Read the model definition and answer for the solid it produces. Units are mm, in the model's axes. Face numbers are marked on the shaded views. A direction names the side the tool comes from. Coordinates: 2 decimals unless noted, no trailing zeros. Write each loop counter-clockwise with the first axis right and the second up, starting at its lowest first coordinate (ties: lowest second). Pieces come first, ordered by that corner, then holes. Notation, with made-up numbers: (77.25, 82) - (120.25, 82) arc R18 cw to (120.25, 103) - close; hole circle Ø2 at (10.5, 40.5). An arc over 180 degrees is marked (long way). Use a Markdown table: item, result.
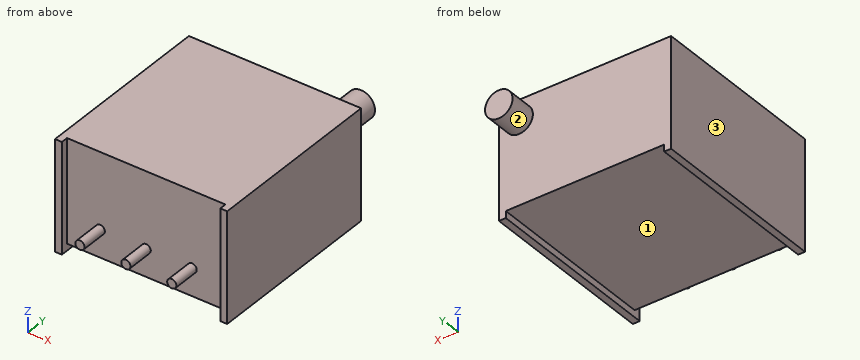
from build123d import *

# Parameters (mm, degrees)
BASE_EXTRUDE_DEPTH = 6.096
SKETCH2_W          = 8.763
SKETCH2_H          = 0.381
CUT_EXTRUDE1_DEPTH = 13.66900593
SKETCH3_R          = 0.762
SCREW_DEPTH        = 1.524
SKETCH4_R          = 0.254
PINS_DEPTH         = 1.524


with BuildPart() as part:
    # Sketch1 → Base-Extrude (new body)
    with BuildSketch(Plane.XY):
        Polygon((4.3815, 0), (4.7625, 0), (4.7625, 10.033), (-4.7625, 10.033), (-4.7625, 0), (-4.3815, 0), (-4.3815, 0.381), (4.3815, 0.381), align=None)
    extrude(amount=-BASE_EXTRUDE_DEPTH)

    # Sketch2 → Cut-Extrude1 (cut, through all)
    with BuildSketch(Plane(origin=(0, 10.033, 0), x_dir=(-1, 0, 0), z_dir=(0, 1, 0))):
        with Locations((0, -5.9055)):
            Rectangle(SKETCH2_W, SKETCH2_H)
    extrude(amount=-CUT_EXTRUDE1_DEPTH, mode=Mode.SUBTRACT)

    # Sketch3 → screw (add)
    with BuildSketch(Plane(origin=(0, 10.033, 0), x_dir=(-1, 0, 0), z_dir=(0, 1, 0))):
        with Locations(Location((-3.6449, -1.0922, 0), (0, 0, 270))):
            Circle(SKETCH3_R)
    extrude(amount=SCREW_DEPTH)

    # Sketch4 → Pins (add)
    with BuildSketch(Plane.XZ.offset(-0.381)):
        with Locations(Location((-2.54, -4.191, 0), (0, 0, 270))):
            Circle(SKETCH4_R)
        with Locations(Location((0, -4.191, 0), (0, 0, 270))):
            Circle(SKETCH4_R)
        with Locations(Location((2.54, -4.191, 0), (0, 0, 270))):
            Circle(SKETCH4_R)
    extrude(amount=PINS_DEPTH)


solid = part.part
(1) Straight lines are drawn through the part: L1, parallel to Y at x = -2.75, z = -1.25; L2, parallel to Z at x = -2, y = 6.25 (3 decimals); L3, parallel to Y at x = 3.5, z = -0.75. For each, find the intervals that lie inside material, in ascending order.
Report:
| item | result |
|---|---|
| L1 | y = 0.38 to 10.03 |
| L2 | z = -5.715 to 0 |
| L3 | y = 0.38 to 11.56 |
(2) For the marked faces 1, 2 and 3, determine the directions among +Z, -Z, +X, -X, +Y, -Y from which every point of the face is accessible in a straight line to the end or side of a thin tool.
Report:
| item | result |
|---|---|
| face 1 | -Z, +Y, -Y |
| face 2 | +Y |
| face 3 | +Z, -Z, -X, +Y, -Y |
(3) A cutting plane is placed at A-A, the plane x = 2.54. Write down the section's boundary in (y, z) (3 decimals).
Report:
| item | result |
|---|---|
| outline | (-1.143, -4.445) - (0.381, -4.445) - (0.381, -5.715) - (10.033, -5.715) - (10.033, 0) - (0.381, 0) - (0.381, -3.937) - (-1.143, -3.937) - close |
(4) A cutting plane is placed at C-C, the plane z = -1. Write down the section's boundary in (x, y).
Report:
| item | result |
|---|---|
| outline | (-4.76, 0) - (-4.38, 0) - (-4.38, 0.38) - (4.38, 0.38) - (4.38, 0) - (4.76, 0) - (4.76, 10.03) - (4.4, 10.03) - (4.4, 11.56) - (2.89, 11.56) - (2.89, 10.03) - (-4.76, 10.03) - close |
(5) This flat-tipped pin is pushed along its axis until it touches: P1, Ø1.5, axis at x = 1.5, z = -2, coming from the +Y side. Where does it stop, or does it pass through?
Report:
| item | result |
|---|---|
| P1 | stops at y = 10.03 |
